Check sheet for the modelled part. Datum: model origin and axes. Units: mm. Face numbers are marked on the shaded views. A direction names the side the tool comes from. Round coordinates to 2 decimals unless told otherwise and drop trailing zeros. Order: outer loops, then holes, each group sorted by start corner. A loop starts at its lowest first (then second) coordinate and runs counter-clockwise, first axis right, second up.
(1) Tool access check on the marked faces 4, 5 and 6. Record the directions out of +Z, -Z, +X, -X, +Y, -Y that give a thin tool (end or side, any length) a straight path to the whole face; none if there is none.
(2) Sectioned sample at B-B, the plane z = 0. Enter the section's corners in (x, y).
(3) Mould release check, pull along Y, two halves, no side actions. Record for the marked faces 1, 2 and 3: released by +Y, released by -Y, zero draft, split by the parting line, or undercut.
(4) Depth check by flat-ended pin: pin 1 (5 mm diameter, centred on x = -1.5, y = 27.5, fed in from +Z) (3 decimals); pin 2 (5 mm diameter, centred on y = 30, z = -19.5, fed in from -X) (3 decimals); pin 3 (4 mm diameter, centred on y = 23, z = -16, fed in from +X) (3 decimals). Enter the tip coordinate at first touch or a pass-through.
(5) Sectioned sample at D-D, the plane y = 17.5. Enter the section's corners in (x, z) (3 decimals), and give its area (3 significant figures).
(6) Sectioned sample at A-A, the plane x = 0. Enter the section's corners in (y, z) (3 decimals).
(7) Sectioned sample at C-C, the plane z = -12.5. Enter the section's corners in (x, y), and give its area (3 significant figures).
(8) Thickness scan on probe 1 along Y at (x, z) = (-1, -19.5); probe 2 along X at (y, z) = (14, 0); probe 3 along Y at (x, z) = (0, -14.5). Record the ranges inside material, lowest first.
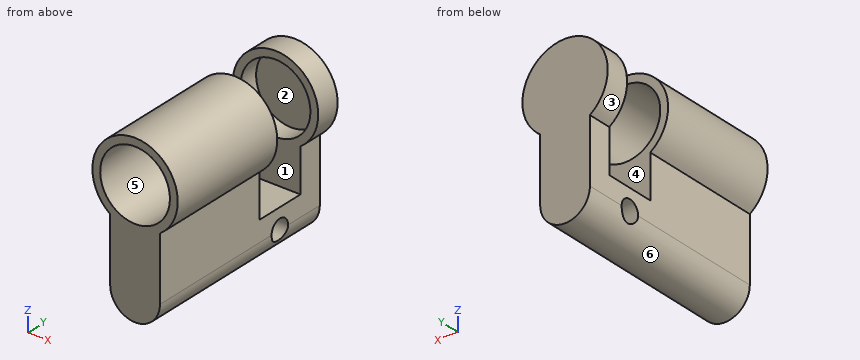
Solid Edge part; units mm, degrees
sketch "Sketch1" plane through (0, 0, 0) normal (0, -1, 0) x (1, 0, 0)
  line L0 (4.925, -19.5) -> (4.925, -6.8664)
  line L1 (-4.925, -19.5) -> (-4.925, -6.8664)
  arc A0 (-4.925, -19.5) -> (4.925, -19.5) centre (0, -19.5) ccw
  arc A1 (4.925, -6.8664) -> (-4.925, -6.8664) centre (0, 0) ccw
extrude "Protrusion1" add sketch "Sketch1" against normal blind 40
sketch "Sketch2" plane through (0, 0, -7.9875) normal (0, -1, 0) x (0, 0, -1)
  circle A0 centre (-7.9875, 0) radius 6.9
extrude "Ausschnitt_1" cut sketch "Sketch2" against normal blind 39
sketch "Sketch3" plane through (0, 0, 0) normal (1, 0, 0) x (0, 1, 0)
  line L0 (35.15, 8.45) -> (24.9, 8.45)
  line L1 (24.9, 8.45) -> (24.9, -15.425)
  line L2 (24.9, -15.425) -> (35.15, -15.425)
  line L3 (35.15, 8.45) -> (35.15, -15.425)
  dimension "D1" = 35.15
extrude "Cutout1" cut sketch "Sketch3" against normal through all and the other way through all
hole "Bohrung_1" at (4.925, 30, -19.5) direction (1, 0, 0) diameter 4.134 end through all both ways yes thread major 5 thread length 2
Derived:
1. face 4: +Z, +X, -X
1. face 5: -Y
1. face 6: -Z, +Y, -Y
2. outline: (-8.45, 0) - (-6.9, 0) - (-6.9, 24.9) - (-8.45, 24.9) - close; (-8.45, 35.15) - (-6.9, 35.15) - (-6.9, 39) - (6.9, 39) - (6.9, 35.15) - (8.45, 35.15) - (8.45, 40) - (-8.45, 40) - close; (6.9, 0) - (8.45, 0) - (8.45, 24.9) - (6.9, 24.9) - close
3. face 1: undercut
3. face 2: released by -Y
3. face 3: zero draft
4. pin 1: stops at z = -15.425
4. pin 2: stops at x = -4.925
4. pin 3: stops at x = 4.925
5. outline: (-4.925, -19.5) arc R4.925 ccw to (4.925, -19.5) - (4.925, -6.866) arc R8.45 ccw (long way) to (-4.925, -6.866) - close; hole circle Ø13.8 at (0, 0)
5. area: 227 mm2
6. outline: (0, -24.425) - (40, -24.425) - (40, 8.45) - (35.15, 8.45) - (35.15, 6.9) - (39, 6.9) - (39, -6.9) - (35.15, -6.9) - (35.15, -15.425) - (24.9, -15.425) - (24.9, -6.9) - (0, -6.9) - close; (0, 6.9) - (24.9, 6.9) - (24.9, 8.45) - (0, 8.45) - close; hole circle Ø4.134 at (30, -19.5)
7. outline: (-4.92, 0) - (4.92, 0) - (4.92, 24.9) - (-4.92, 24.9) - close; (-4.92, 35.15) - (4.92, 35.15) - (4.92, 40) - (-4.92, 40) - close
7. area: 293 mm2
8. probe 1: y = 0 to 27.93, 32.07 to 40
8. probe 2: x = -8.45 to -6.9, 6.9 to 8.45
8. probe 3: y = 0 to 24.9, 35.15 to 40
